Check sheet for the modelled part. Datum: model origin and axes. Units: mm. A direction names the side the tool comes from. Give positions to 0.01 mm unless a question says otherwise; leave off trailing zeros. Use CSV: the item, a comma, the result in double quotes.
Autodesk Inventor part; units mm, degrees
ref_plane "Work Plane3" through (0, 0, 0) normal (0, -0.7071, 0.7071) x (1, 0, 0)
ref_plane "YZ Plane" through (0, 0, 0) normal (1, 0, 0) x (0, 1, 0)
ref_plane "XZ Plane" through (0, 0, 0) normal (0, 1, 0) x (-1, 0, 0)
sketch "Sketch1" plane through (0, 0, 0) normal (0, 0, 1) x (1, 0, 0)
  circle A0 centre (0, 0) radius 100 construction
  circle A1 centre (0, 0) radius 75 construction
  circle A2 centre (0, 75) radius 24 construction
  circle A3 centre (0, 0) radius 89 construction
  dimension "d8" = 150
  dimension "d7" = 200
  dimension "d9" = 48
  dimension "d10" = 14
sketch "Sketch6" plane through (0, 0, 0) normal (0, 0, 1) x (1, 0, 0)
  point P0 (0, 0)
ref_plane "Work Plane3" through (0, 0, 0) normal (0, -0.7071, 0.7071) x (1, 0, 0)
sketch "2d Roller Ellipse" plane through (0, 0, 0) normal (0, -0.7071, 0.7071) x (1, 0, 0)
  ellipse E0 centre (0, 0) end of major axis (100, 0) minor radius 70.7107 construction
  ellipse E1 centre (0, 53.033) end of major axis (24, 53.033) minor radius 16.9706 construction
  ellipse E2 centre (0, 0) end of major axis (100, 0) minor radius 70.7107 construction
  ellipse E3 centre (0, 0) end of major axis (-100, 0) minor radius 70.0036 construction
  line L0 (0, 70.0036) -> (0, 67.0036) construction
  line L1 (0, 67.0036) -> (0, 46.0036) construction
  circle A0 centre (0, 46.0036) radius 21 construction
  ellipse E4 centre (0, 0) end of major axis (-97, 0) minor radius 67.0036 (47.2844, 58.5036) -> (-47.2844, 58.5036) ccw
  line L2 (0, 46.0036) -> (0, 58.5036) construction
  line L3 (0, 58.5036) -> (51.8941, 58.5036) construction
  line L4 (47.2844, 58.5036) -> (47.2844, 46.0036)
  line L5 (47.2844, 46.0036) -> (0, 46.0036)
  line L6 (-47.2844, 58.5036) -> (-47.2844, 46.0036)
  line L7 (-47.2844, 46.0036) -> (0, 46.0036)
  dimension "d53" = 25
  dimension "d61" = 100
  dimension "d63" = 70.7107
  dimension "d77" = 3
  dimension "d78" = 21
  dimension "d79" = 42
  dimension "d80" = 12.5
  dimension "d81" = 12.5
  dimension "d82" = 4.6098
revolve "Revolution4" add sketch "2d Roller Ellipse" angle 360 about axis through (-47.2844, 32.5294, 32.5294) along (1, 0, 0)
sketch "Sketch11" plane through (47.2844, 32.5294, 32.5294) normal (1, 0, 0) x (0, 0, -1)
  circle A0 centre (0, 0) radius 12.5
  point P0 (32.5294, -32.5294)
  point P1 (-8.8388, 8.8388)
hole "Hole1" at (47.2844, 32.5294, 32.5294) direction (-1, 0, 0) diameter 6 end through all
sketch "Sketch12" plane through (47.2844, 32.5294, 32.5294) normal (1, 0, 0) x (0, 0, -1)
  circle A0 centre (0, 0) radius 11
  circle A1 centre (0, 0) radius 12.5
  point P0 (32.5294, -32.5294)
  point P1 (-8.8388, 8.8388)
  dimension "d93" = 22
extrude "Extrusion5" cut sketch "Sketch12" against normal blind 8 contours A0
sketch "Sketch13" plane through (-47.2844, 32.5294, 32.5294) normal (-1, 0, 0) x (0, 0, 1)
  circle A0 centre (0, 0) radius 12.5
  circle A1 centre (0, 0) radius 3
  circle A2 centre (0, 0) radius 11
  point P0 (-32.5294, -32.5294)
  point P1 (8.8388, 8.8388)
  dimension "d96" = 22
extrude "Extrusion6" cut sketch "Sketch13" against normal blind 8 contours A2
properties part number "Mecanum_Roller_48mm"
1. Set-up check for faces 1 (the face through (-0.55, 30, 30.92)), 2 (the face through (-39.284, 30, 35)), 3 (the face through (43.34, 21.79, 34.91)): record each of +Z, -Z, +X, -X, +Y, -Y from which the full face is reachable in a straight line by a thin tool's end or side.
Completed:
face 1,"+X, -X"
face 2,"-X"
face 3,"+X"
2. Release check for a two-part mould opening along Y. For faces 4 (the face through (39.284, 30, 30)), 5 (the face through (-47.284, 41, 25)) record: released by +Y, released by -Y, zero draft, split by the parting line, or undercut.
Completed:
face 4,"undercut"
face 5,"zero draft"
3. Scan lines: line 1 along X through (y, z) = (37, 37.5); line 2 along Z through (x, y) = (30.5, 34); line 3 along Y through (x, z) = (22.5, 34.5). Record each from-to range of solid material in increasing order.
Completed:
line 1,"x = -39.28 to 39.28"
line 2,"z = 14.99 to 29.91, 35.14 to 50.07"
line 3,"y = 13.46 to 30.27, 34.79 to 51.6"
4. Go/stop test with flat-tipped pins: pin 1 Ø20 at (y, z) = (32.53, 32.53) entering from -X; pin 2 Ø1.5 at (y, z) = (37.5, 24.5) entering from +X; pin 3 Ø1.5 at (x, y) = (0, 34) entering from -Z. Record where each tip stops, or that it passes through.
Completed:
pin 1,"stops at x = -39.28"
pin 2,"stops at x = 39.28"
pin 3,"stops at z = 11.54"
